```python
from build123d import *

# Parameters (mm, degrees)
F0_W     = 100
F0_H     = 25
F1_DEPTH = 10
F2_W     = 30
F2_H     = 25
F3_DEPTH = 50
F4_W     = 15.893344
F4_H     = 13.28928
F5_DEPTH = 25.001
F7_DEPTH = 25


with BuildPart() as f1:
    # F0 (on Top) → F1 (new body)
    with BuildSketch(Plane.XY):
        with Locations((14.104442, 41.370601)):
            Rectangle(F0_W, F0_H)
    extrude(amount=F1_DEPTH)

    # F2 (on face) → F3 (join)
    with BuildSketch(Plane.XY.offset(10)):
        with Locations((49.104442, 41.370601)):
            Rectangle(F2_W, F2_H)
    extrude(amount=F3_DEPTH)

    # F4 (on face) → F5 (cut, through all)
    with BuildSketch(Plane.XZ.offset(-28.870601)):
        with Locations((49.347391, 43.861993)):
            Rectangle(F4_W, F4_H)
    extrude(amount=-F5_DEPTH, mode=Mode.SUBTRACT)

    # F6 (on face) → F7 (cut)
    with BuildSketch(Plane.XY.offset(10)):
        with BuildLine():
            Line((-22.895558, 41.051087), (24.104442, 41.051087))
            Line((24.104442, 41.051087), (24.104442, 47.251087))
            Line((24.104442, 47.251087), (-22.895558, 47.251087))
            ThreePointArc((-22.895558, 47.251087), (-25.016878, 46.372407), (-25.895558, 44.251087))
            Line((-25.895558, 44.251087), (-25.895558, 44.051087))
            ThreePointArc((-25.895558, 44.051087), (-25.016878, 41.929766), (-22.895558, 41.051087))
        make_face()
    extrude(amount=-F7_DEPTH, mode=Mode.SUBTRACT)


solid = f1.part
```
Geometry check sheet. Reference: the model listing, model coordinates, mm. A direction names the side the tool comes from. Give positions to 0.01 mm unless a question says otherwise; leave off trailing zeros. Loops run counter-clockwise (first coordinate to the right, second up) from the corner with the lowest first, then second, coordinate; pieces in that order, holes last. Notation, with made-up numbers: M 66,72.25 L 94,72.25 A20 ccw 94,84.25 Z; hole C 61,-12 d2. An arc over 180 degrees is marked long. Answer as CSV lines item,"result".
Item 1: Access from +Z, -Z, +X, -X, +Y, -Y to the whole of each face (thin tool, end or side, straight path). Record for faces 4 (the flat face through (-1, 39, 10)), 5 (the flat face through (49, 41, 37.217)), 6 (the flat face through (-35.896, 41, 5)), 7 (the cylindrical face through (-24.99, 46.4, 5.07)).
Values:
face 4,"+Z, -X, +Y, -Y"
face 5,"+Y, -Y"
face 6,"+Z, -Z, -X, +Y, -Y"
face 7,"+Z, -Z"
Item 2: Cross-section at C-C on x = -20. Record the cut outline in (y, z).
Values:
outline,"M 28.87,0 L 41.05,0 L 41.05,10 L 28.87,10 Z; M 47.25,0 L 53.87,0 L 53.87,10 L 47.25,10 Z"
Item 3: Depth check by flat-ended pin: P1, Ø8, axis at y = 37, z = 19, coming from the -X side; P2, Ø7.5, axis at x = -9.5, y = 42.5, coming from the +Z side. Enter the tip coordinate at first touch or a pass-through.
Values:
P1,"stops at x = 34.1"
P2,"stops at z = 10"
Item 4: Cross-section at D-D on z = 8.5. Record the cut outline in (x, y).
Values:
outline,"M -35.9,28.87 L 64.1,28.87 L 64.1,53.87 L -35.9,53.87 Z; hole M -25.9,44.05 A3 ccw -22.9,41.05 L 24.1,41.05 L 24.1,47.25 L -22.9,47.25 A3 ccw -25.9,44.25 Z"
Item 5: Release check for a two-part mould opening along X. For faces 1 (the flat face through (49, 42, 60)), 2 (the flat face through (57.294, 41, 44)), 3 (the flat face through (64.104, 41, 30)) record: pulls with the +X half, pulls with the -X half, needs draft (parallel to the pull), parting line crosses it, or undercut.
Values:
face 1,"needs draft"
face 2,"undercut"
face 3,"pulls with the +X half"
Item 6: Material ranges on line 1 (Z direction, x = 56.5, y = 45.5); line 2 (Z direction, x = -8.5, y = 32); line 3 (X direction, y = 45, z = 30), recorded low to high.
Values:
line 1,"z = 0 to 37.22, 50.51 to 60"
line 2,"z = 0 to 10"
line 3,"x = 34.1 to 64.1"
Item 7: Cross-section at A-A on z = 41. Record the cut outline in (x, y).
Values:
outline,"M 34.1,28.87 L 41.4,28.87 L 41.4,53.87 L 34.1,53.87 Z; M 57.29,28.87 L 64.1,28.87 L 64.1,53.87 L 57.29,53.87 Z"
Item 8: Cross-section at B-B on y = 31.5. Record the cut outline in (x, z), and give its area (3 significant figures).
Values:
outline,"M -35.9,0 L 64.1,0 L 64.1,60 L 34.1,60 L 34.1,10 L -35.9,10 Z; hole M 41.4,37.22 L 57.29,37.22 L 57.29,50.51 L 41.4,50.51 Z"
area,"2,290 mm²"
